Source: CAD feature listing. Evaluate the final solid. Frame: model axes, mm. A direction names the side the tool comes from. Give positions to 0.01 mm unless a question says otherwise; leave off trailing zeros. Order: outer loops, then holes, each group sorted by start corner. A loop starts at its lowest first (then second) coordinate and runs counter-clockwise, first axis right, second up.
from build123d import *

# Parameters (mm, degrees)
SKETCH1_R           = 30.1
BOSS_EXTRUDE1_DEPTH = 10
SKETCH1_3_R         = 2.5
BOSS_EXTRUDE2_DEPTH = 10


with BuildPart() as part:
    # Sketch1 → Boss-Extrude1 (new body)
    with BuildSketch(Plane.XY):
        Circle(SKETCH1_R)
    extrude(amount=BOSS_EXTRUDE1_DEPTH)

    # Sketch1<3> → Boss-Extrude2 (add)
    with BuildSketch(Plane.XY):
        with Locations((0, 12.5)):
            Circle(SKETCH1_3_R)
        with Locations((-9.013601894, -8.660541605)):
            Circle(SKETCH1_3_R)
        with Locations((9.013601894, -8.660541605)):
            Circle(SKETCH1_3_R)
    extrude(amount=-BOSS_EXTRUDE2_DEPTH)


solid = part.part
1) Ray query, L1, parallel to Z at x = -16, y = -20.5; L2, parallel to X at y = 0.5, z = 6.75. Return the intervals inside material, ascending.
Checks:
L1: z = 0 to 10
L2: x = -30.1 to 30.1
2) Reachability of faces 1 (the face through (-0.54, 10.06, -4.93)), 2 (the face through (9, -9, -10)) from +Z, -Z, +X, -X, +Y, -Y: full face, straight path, thin tool, end or side. Return the list, or none.
Checks:
face 1: -Z
face 2: -Z, +X, -X, +Y, -Y
3) Pull-direction query (X, two-part tool) for faces 3 (the face through (0, 13, -10)), 4 (the face through (-9.34, -6.18, -4.93)), 5 (the face through (-6.525, -29.384, 4.93)); classes: +X half, -X half, draft (parallel to the pull), parting line (faces both ways), or undercut.
Checks:
face 3: draft
face 4: undercut
face 5: parting line
4) Section query B-B on y = 12.5. Output: boundary loops of the cut face in (x, z).
Checks:
outline: (-27.38, 0) - (-2.5, 0) - (-2.5, -10) - (2.5, -10) - (2.5, 0) - (27.38, 0) - (27.38, 10) - (-27.38, 10) - close
5) First-contact query: pin 1 Ø1.5 at (x, z) = (6.5, -4) entering from -Y; pin 2 Ø1 at (y, z) = (-7, -7.5) entering from +X; pin 3 Ø10 at (x, z) = (17.5, -4) entering from -Y; pin 4 Ø2 at (x, z) = (4.5, -2.5) entering from +Y. Flat tips, straight axial feed; report the tip coordinate or a pass-through.
Checks:
pin 1: stops at y = -10.43
pin 2: stops at x = 11.23
pin 3: stops at y = -26.38
pin 4: passes through
6) Section query C-C on z = 2. Output: boundary loops of the cut face in (x, y), and give its area (3 significant figures).
Checks:
outline: circle Ø60.2 at (0, 0)
area: 2,850 mm2
7) Section query A-A on x = 0. Output: boundary loops of the cut face in (y, z).
Checks:
outline: (-30.1, 0) - (10, 0) - (10, -10) - (15, -10) - (15, 0) - (30.1, 0) - (30.1, 10) - (-30.1, 10) - close
8) Section query D-D on y = 0. Output: boundary loops of the cut face in (x, z).
Checks:
outline: (-30.1, 0) - (30.1, 0) - (30.1, 10) - (-30.1, 10) - close
